Source: CAD feature listing. Evaluate the final solid. Frame: model axes, mm. Face numbers are marked on the shaded views. A direction names the side the tool comes from. Give positions to 0.01 mm unless a question says otherwise; leave off trailing zeros. Write each loop counter-clockwise with the first axis right and the second up, starting at its lowest first coordinate (ties: lowest second). Pieces come first, ordered by that corner, then holes. Notation, with made-up numbers: (75, -12.75) -> (121, -12.75) arc R37 ccw to (121, 25.25) -> close; hole circle Ø2 at (83.25, 33.5). An arc over 180 degrees is marked (long way). Use a Markdown table: item, result. Add a question column.
```python
from build123d import *

# Parameters (mm, degrees)
F1_DEPTH = 35
F3_DEPTH = 10
F5_DEPTH = 35
F6_R     = 2.5


with BuildPart() as f1:
    # F0 (on Top) → F1 (new body)
    with BuildSketch(Plane.XY):
        Polygon((-20, 13.5), (-20, 11), (20, 11), (20, -11), (-20, -11), (-20, -13.5), (22.5, -13.5), (22.5, 13.5), align=None)
    extrude(amount=F1_DEPTH)

    # F2 (on face) → F3 (join)
    with BuildSketch(Plane(origin=(0, 0, 0), x_dir=(1, 0, 0), z_dir=(0, 0, -1))):
        Polygon((-19, -11), (-13, -11), (-13, -8), (-19, -10), align=None)
    extrude(amount=-F3_DEPTH)

    # F4 (on face) → F5 (join)
    with BuildSketch(Plane(origin=(0, 0, 0), x_dir=(1, 0, 0), z_dir=(0, 0, -1))):
        Polygon((-20, -13.5), (-20, -11), (-23.267881, -13.694357), (-21.817495, -15.453473), (-19.448203, -13.5), align=None)
    extrude(amount=-F5_DEPTH)

    # F6
    f6_edges = [f1.edges().sort_by_distance(p)[0] for p in [
        (22.5, 13.5, 17.5),
        (22.5, -13.5, 17.5),
    ]]
    fillet(f6_edges, radius=F6_R)


solid = f1.part
```
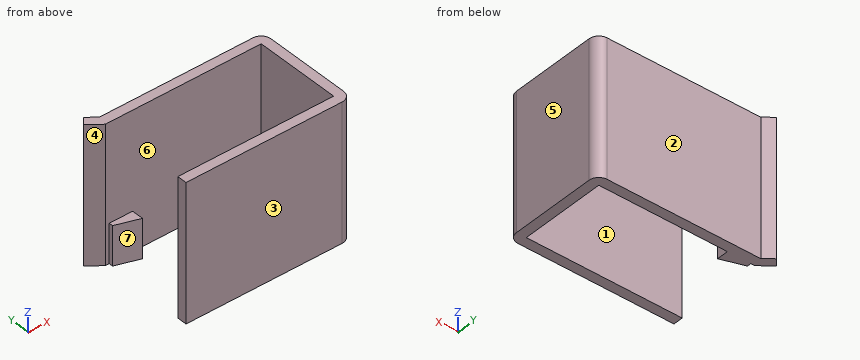
(1) Cut plane B-B on z = 32.5. Return the cut outline in (x, y).
(2) First-contact query: pin 1 Ø1.5 at (x, z) = (16, 18) entering from +Y; pin 2 Ø2.5 at (x, y) = (-16, 9.5) entering from +Z; pin 3 Ø11 at (y, z) = (2.5, 18.5) entering from -X. Flat tips, straight axial feed; report the tip coordinate or a pass-through.
(3) Mould query, pull axis Y, two halves, no side actions, for the marked faces 4, 5, 6 and 7. Classes: +Y half, -Y half, draft (parallel to the pull), parting line (faces both ways), or undercut.
(4) Access query for the marked faces 1, 2 and 3. Directions: +Z, -Z, +X, -X, +Y, -Y. A direction counts if a zero-diameter tool reaches every point of the face in a straight line with its end or side. Return the directions, or none.
(5) Cut plane C-C on y = 2.75. Return the cut outline in (x, z).
(6) Cut plane D-D on z = 7. Return the cut outline in (x, y).
(7) Cut plane A-A on x = 8.5. Return the cut outline in (y, z), then the cut area to 3 significant figures.
(8) Material intervals for L1, parallel to Y at x = 2, z = 22; L2, parallel to X at y = -0.25, z = 31.5; L3, parallel to Y at x = -18, z = 8, sorted ascending.
Output:
| question | item | result |
|---|---|---|
| 1 | outline | (-23.27, 13.69) -> (-20, 11) -> (20, 11) -> (20, -11) -> (-20, -11) -> (-20, -13.5) -> (20, -13.5) arc R2.5 ccw to (22.5, -11) -> (22.5, 11) arc R2.5 ccw to (20, 13.5) -> (-19.45, 13.5) -> (-21.82, 15.45) -> close |
| 2 | pin 1 | y = 13.5 |
| 2 | pin 2 | z = 10 |
| 2 | pin 3 | x = 20 |
| 3 | face 4 | -Y half |
| 3 | face 5 | draft |
| 3 | face 6 | undercut |
| 3 | face 7 | undercut |
| 4 | face 1 | +Z, -Z, -X |
| 4 | face 2 | +Z, -Z, +X, +Y |
| 4 | face 3 | +Z, -Z, +X, -X, -Y |
| 5 | outline | (20, 0) -> (22.5, 0) -> (22.5, 35) -> (20, 35) -> close |
| 6 | outline | (-23.27, 13.69) -> (-20, 11) -> (-19, 11) -> (-19, 10) -> (-13, 8) -> (-13, 11) -> (20, 11) -> (20, -11) -> (-20, -11) -> (-20, -13.5) -> (20, -13.5) arc R2.5 ccw to (22.5, -11) -> (22.5, 11) arc R2.5 ccw to (20, 13.5) -> (-19.45, 13.5) -> (-21.82, 15.45) -> close |
| 7 | outline | (-13.5, 0) -> (-11, 0) -> (-11, 35) -> (-13.5, 35) -> close; (11, 0) -> (13.5, 0) -> (13.5, 35) -> (11, 35) -> close |
| 7 | area | 175 mm^2 |
| 8 | L1 | -13.5 to -11, 11 to 13.5 |
| 8 | L2 | 20 to 22.5 |
| 8 | L3 | -13.5 to -11, 9.67 to 13.5 |
